from build123d import *

# Parameters (mm, degrees)
SKETCH1_R           = 7.5
BOSS_EXTRUDE1_DEPTH = 157.5
SKETCH2_W           = 20
SKETCH2_H           = 20
BOSS_EXTRUDE2_DEPTH = 10
SKETCH3_W           = 20
SKETCH3_H           = 20
BOSS_EXTRUDE3_DEPTH = 10


with BuildPart() as part:
    # Sketch1 → Boss-Extrude1 (new body)
    with BuildSketch(Plane.XY):
        Circle(SKETCH1_R)
    extrude(amount=BOSS_EXTRUDE1_DEPTH)

    # Sketch2 → Boss-Extrude2 (add)
    with BuildSketch(Plane.XY.offset(107.5)):
        Rectangle(SKETCH2_W, SKETCH2_H)
    extrude(amount=BOSS_EXTRUDE2_DEPTH)

    # Sketch3 → Boss-Extrude3 (add)
    with BuildSketch(Plane.XY.offset(32.5)):
        Rectangle(SKETCH3_W, SKETCH3_H)
    extrude(amount=BOSS_EXTRUDE3_DEPTH)


solid = part.part
Design review of the part built by this model. Coordinates are the model's own, in mm. A direction names the side the tool comes from. Round coordinates to 2 decimals unless told otherwise and drop trailing zeros. Write each loop counter-clockwise with the first axis right and the second up, starting at its lowest first coordinate (ties: lowest second). Pieces come first, ordered by that corner, then holes.
Item 1: Consider section A-A on x = -6. Give the boundary of the cut face in (y, z), and give its area (3 significant figures).
Item 2: Draft analysis for pull direction Z (two halves, no side actions). For faces 1 (the flat face through (4, 7, 32.5)), 2 (the flat face through (4, 7, 42.5)), 3 (the flat face through (10, 0, 112)), 4 (the flat face through (4, 7, 107.5)), state which applies: released by +Z, released by -Z, zero draft, split by the parting line, or undercut.
Item 3: For pin 1 Ø10 at (y, z) = (2, 57) entering from -X; pin 2 Ø8 at (x, z) = (-2.5, 48) entering from -Y; pin 3 Ø2 at (x, z) = (4, 72.5) entering from -Y, all flat-tipped, find the tip position at first contact; note any pin that passes through.
Item 4: For faces 5 (the flat face through (4, 7, 117.5)), 6 (the cylindrical face through (-7.493, 0.33, 74.545)), 7 (the cylindrical face through (-7.493, 0.33, 16.022)), 8 (the flat face through (0, -10, 37)), list the 3-axis set-ups (+Z, -Z, +X, -X, +Y, -Y) from which the entire face can be reached by the end or side of a thin tool; tool diameter is ignored.
Item 5: Wall thickness on L1, parallel to Z at x = -5.25, y = -5.75; L2, parallel to X at y = -0.5, z = 132.5; L3, parallel to Y at x = -6.5, z = 121.5: over which ranges is each line inside the solid? List them lowest first.
Item 6: Consider section B-B on y = 0. Give the boundary of the cut face in (x, z).
Item 7: Consider section C-C on z = 84. Give the boundary of the cut face in (x, y).
Check values:
1. outline: (-10, 32.5) - (-4.5, 32.5) - (-4.5, 0) - (4.5, 0) - (4.5, 32.5) - (10, 32.5) - (10, 42.5) - (4.5, 42.5) - (4.5, 107.5) - (10, 107.5) - (10, 117.5) - (4.5, 117.5) - (4.5, 157.5) - (-4.5, 157.5) - (-4.5, 117.5) - (-10, 117.5) - (-10, 107.5) - (-4.5, 107.5) - (-4.5, 42.5) - (-10, 42.5) - close
1. area: 1,640 mm2
2. face 1: released by -Z
2. face 2: undercut
2. face 3: zero draft
2. face 4: undercut
3. pin 1: stops at x = -7.5
3. pin 2: stops at y = -7.5
3. pin 3: stops at y = -6.87
4. face 5: +Z
4. face 6: none
4. face 7: -Z
4. face 8: +Z, -Z, +X, -X, -Y
5. L1: z = 32.5 to 42.5, 107.5 to 117.5
5. L2: x = -7.48 to 7.48
5. L3: y = -3.74 to 3.74
6. outline: (-10, 32.5) - (-7.5, 32.5) - (-7.5, 0) - (7.5, 0) - (7.5, 32.5) - (10, 32.5) - (10, 42.5) - (7.5, 42.5) - (7.5, 107.5) - (10, 107.5) - (10, 117.5) - (7.5, 117.5) - (7.5, 157.5) - (-7.5, 157.5) - (-7.5, 117.5) - (-10, 117.5) - (-10, 107.5) - (-7.5, 107.5) - (-7.5, 42.5) - (-10, 42.5) - close
7. outline: circle Ø15 at (0, 0)
